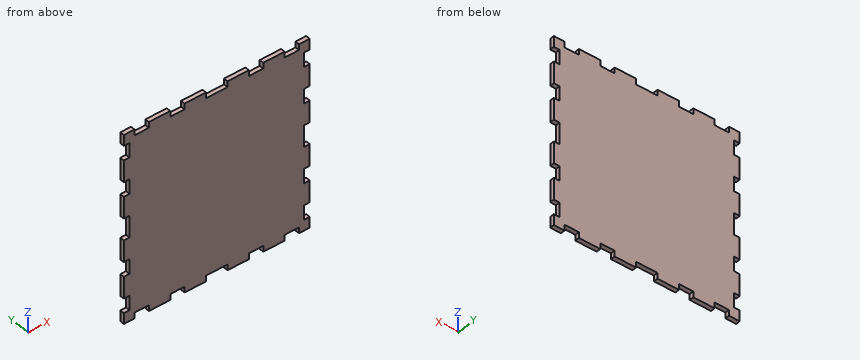
from build123d import *

# Parameters (mm, degrees)
BOSS_EXTRUDE1_DEPTH = 3


with BuildPart() as part:
    # Sketch1 → Boss-Extrude1 (new body)
    with BuildSketch(Plane(origin=(0, 0, 0), x_dir=(1, 0, 0), z_dir=(0, 1, 0))):
        Polygon((-65, -65), (-57.5, -65), (-57.5, -61), (-47.5, -61), (-47.5, -65), (-32.5, -65), (-32.5, -61), (-22.5, -61), (-22.5, -65), (-7.5, -65), (-7.5, -61), (7.5, -61), (7.5, -65), (22.5, -65), (22.5, -61), (32.5, -61), (32.5, -65), (47.5, -65), (47.5, -61), (57.5, -61), (57.5, -65), (65, -65), (65, -57.5), (61, -57.5), (61, -47.5), (65, -47.5), (65, -32.5), (61, -32.5), (61, -22.5), (65, -22.5), (65, -7.5), (61, -7.5), (61, 7.5), (65, 7.5), (65, 22.5), (61, 22.5), (61, 32.5), (65, 32.5), (65, 47.5), (61, 47.5), (61, 57.5), (65, 57.5), (65, 65), (57.5, 65), (57.5, 61), (47.5, 61), (47.5, 65), (32.5, 65), (32.5, 61), (22.5, 61), (22.5, 65), (7.5, 65), (7.5, 61), (-7.5, 61), (-7.5, 65), (-22.5, 65), (-22.5, 61), (-32.5, 61), (-32.5, 65), (-47.5, 65), (-47.5, 61), (-57.5, 61), (-57.5, 65), (-65, 65), (-65, 57.5), (-61, 57.5), (-61, 47.5), (-65, 47.5), (-65, 32.5), (-61, 32.5), (-61, 22.5), (-65, 22.5), (-65, 7.5), (-61, 7.5), (-61, -7.5), (-65, -7.5), (-65, -22.5), (-61, -22.5), (-61, -32.5), (-65, -32.5), (-65, -47.5), (-61, -47.5), (-61, -57.5), (-65, -57.5), align=None)
    extrude(amount=BOSS_EXTRUDE1_DEPTH)


solid = part.part
Build history of the part. All positions in model axes, mm. Coordinates: 2 decimals unless noted, no trailing zeros. Order: outer loops, then holes, each group sorted by start corner. A loop starts at its lowest first (then second) coordinate and runs counter-clockwise, first axis right, second up. Notation, with made-up numbers: M 35,87.5 L 62,87.5 A17 ccw 62,92.5 Z; hole C 89,30.5 d3. An arc over 180 degrees is marked long. One line per question, with ' | ' between items. Start each with the question number.
Q1. Probe L1, parallel to X at y = 1.45, z = -25. List the from-to ranges inside material, lowest first. Write a range as from..to.
Q2. Saw through at A-A (x = 3). List the corners of the cut face in (y, z).
Q3. Flat gauge pins, fed straight in: pin 1 Ø0.9 at (x, y) = (-54.5, 2) entering from -Z; pin 2 Ø1 at (y, z) = (1, -2.5) entering from +X; pin 3 Ø1.5 at (y, z) = (1, 26) entering from -X; pin 4 Ø2 at (x, z) = (-15, 21.5) entering from -Y. Where does each tip first touch, or does it go through?
Check values:
1) L1: x = -61..61
2) outline: M 0,-61 L 3,-61 L 3,61 L 0,61 Z
3) pin 1: stops at z = -61 | pin 2: stops at x = 61 | pin 3: stops at x = -61 | pin 4: stops at y = 0
